Part model, mm, in its own coordinate system. Round coordinates to 2 decimals unless told otherwise and drop trailing zeros. Order: outer loops, then holes, each group sorted by start corner. A loop starts at its lowest first (then second) coordinate and runs counter-clockwise, first axis right, second up. Notation, with made-up numbers: (-10, 70.5) -> (18, 70.5) arc R13 cw to (18, 89.5) -> close; hole circle Ø3 at (59, 61.5). An arc over 180 degrees is marked (long way). Return JSON: item names as keys, results as strings. Group by question number.
from build123d import *

# Parameters (mm, degrees)
SKETCH1_R           = 1.9
BOSS_EXTRUDE1_DEPTH = 5
SKETCH2_R           = 2.5
BOSS_EXTRUDE2_DEPTH = 5


with BuildPart() as part:
    # Sketch1 → Boss-Extrude1 (new body)
    with BuildSketch(Plane.XY):
        with BuildLine():
            Line((13.1, 0), (6, 48.912409848))
            ThreePointArc((6, 48.912409848), (10, 52.912409848), (14, 48.912409848))
            Line((14, 48.912409848), (20.934913045, 1.137295889))
            ThreePointArc((20.934913045, 1.137295889), (17.674607614, -3.958513116), (13.1, 0))
        make_face()
        with Locations((17.1, 0)):
            Circle(SKETCH1_R, mode=Mode.SUBTRACT)
    extrude(amount=BOSS_EXTRUDE1_DEPTH)

    # Sketch2 → Boss-Extrude2 (add)
    with BuildSketch(Plane(origin=(0, 0, 0), x_dir=(-1, 0, 0), z_dir=(0, 0, -1))):
        with Locations(Location((-10, 48.912409848, 0), (0, 0, 180))):
            Circle(SKETCH2_R)
    extrude(amount=BOSS_EXTRUDE2_DEPTH)


solid = part.part
(1) Saw through at C-C, the plane x = 11.25. List the corners of the cut face in (y, z).
(2) Mould opens along Y. For faces 1 (the flat face through (9.6, 24.1, 2.5)), 2 (the cylindrical face through (18.912, 0.571, 2.465)), 3 (the cylindrical face through (9.458, 51.353, -2.465)) say: pulls with the +Y half, pulls with the -Y half, needs draft (parallel to the pull), parting line crosses it, or undercut.
(3) Saw through at A-A, the plane z = 2.5. List the corners of the cut face in (x, y), and give its area (3 significant figures).
(4) Probe L1, parallel to Z at x = 11.75, y = 45; L2, parallel to X at y = 7, z = 3.25; L3, parallel to X at y = 40, z = 1. List the from-to ranges inside material, lowest first. Write a range as [from, to].
(5) Pin check, flat tips, straight feed: P1, Ø4, axis at y = 2, z = -1.5, coming from the -X side; P2, Ø6, axis at y = 22, z = -1.5, coming from the -X side; P3, Ø2.5, axis at x = 17.1, y = 0, coming from the +Z side; P4, Ø7.5, axis at x = 11.5, y = 21.5, coming from the -Z side. Stop position of each tip, or through.
(6) Saw through at B-B, the plane x = 17.5. List the corners of the cut face in (y, z).
(7) Saw through at D-D, the plane z = -0.5. List the corners of the cut face in (x, y).
Results are:
{
 "1": {"outline": "(12.74, 0) -> (46.75, 0) -> (46.75, -5) -> (51.08, -5) -> (51.08, 0) -> (52.71, 0) -> (52.71, 5) -> (12.74, 5) -> close"},
 "2": {"face 1": "pulls with the -Y half", "face 2": "undercut", "face 3": "parting line crosses it"},
 "3": {"outline": "(6, 48.91) -> (13.1, 0) arc R4 ccw (long way) to (20.93, 1.14) -> (14, 48.91) arc R4 ccw to start; hole circle Ø3.8 at (17.1, 0)", "area": "430 mm^2"},
 "4": {"L1": "z = [0, 5]", "L2": "x = [12.08, 20.08]", "L3": "x = [7.29, 15.29]"},
 "5": {"P1": "stops at x = 12.62", "P2": "stops at x = 9.53", "P3": "passes through", "P4": "stops at z = 0"},
 "6": {"outline": "(-3.98, 0) -> (-1.86, 0) -> (-1.86, 5) -> (-3.98, 5) -> close; (1.86, 0) -> (24.8, 0) -> (24.8, 5) -> (1.86, 5) -> close"},
 "7": {"outline": "circle Ø5 at (10, 48.91)"}
}
